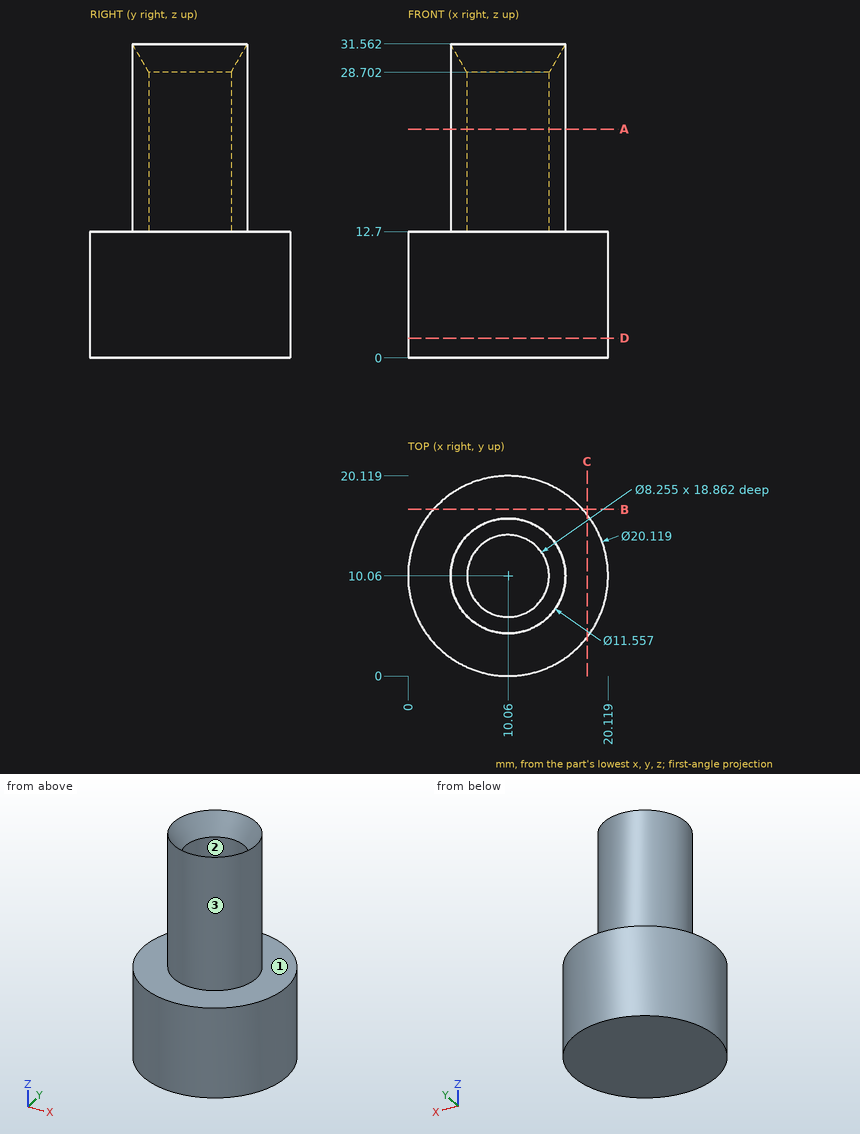
Geometry check sheet. Reference: drawing and pictorial views, mm from the part's lowest x, y, z. Round coordinates to 2 decimals unless told otherwise and drop trailing zeros. Loops run counter-clockwise (first coordinate to the right, second up) from the corner with the lowest first, then second, coordinate; pieces in that order, holes last. Notation, with made-up numbers: (44, 27.25) -> (56, 27.25) arc R33 cw to (56, 58.25) -> close; hole circle Ø9 at (-5, 19.25). An arc over 180 degrees is marked (long way). Use a Markdown table: item, result.
(1) Sectioned sample at B-B (y = 16.75). Enter the section's corners in (x, z), then the cut area to 3 significant figures.
Calculated:
| item | result |
|---|---|
| outline | (2.55, 0) -> (17.57, 0) -> (17.57, 12.7) -> (2.55, 12.7) -> close |
| area | 191 mm² |
(2) Go/stop test with flat-tipped pins: P1, Ø6.5, axis at x = 11, y = 8, coming from the +Z side (1 decimal); P2, Ø1, axis at y = 13, z = 20.5, coming from the -X side; P3, Ø2, axis at y = 5.5, z = 7, coming from the +X side. Record where each tip stops, or that it passes through.
Calculated:
| item | result |
|---|---|
| P1 | z = 31.1 |
| P2 | x = 4.82 |
| P3 | x = 19.47 |
(3) Sectioned sample at A-A (z = 23). Enter the section's corners in (x, y) (1 decimal).
Calculated:
| item | result |
|---|---|
| outline | circle Ø11.6 at (10.1, 10.1); hole circle Ø8.3 at (10.1, 10.1) |
(4) Scan lines: probe 1 along Z at (x, y) = (5.5, 1.25); probe 2 along Y at (x, z) = (8.25, 23); probe 3 along X at (y, z) = (7.25, 25.5) (1 decimal). Record each from-to range of solid material in increasing order.
Calculated:
| item | result |
|---|---|
| probe 1 | 0 to 12.7 |
| probe 2 | 4.57 to 6.35, 13.77 to 15.55 |
| probe 3 | 5 to 7, 13.1 to 15.1 |
(5) Mould release check, pull along Y, two halves, no side actions. Record for the marked faces 1, 2 and 3: released by +Y, released by -Y, zero draft, split by the parting line, or undercut.
Calculated:
| item | result |
|---|---|
| face 1 | zero draft |
| face 2 | undercut |
| face 3 | split by the parting line |
(6) Sectioned sample at D-D (z = 2). Enter the section's corners in (x, y).
Calculated:
| item | result |
|---|---|
| outline | circle Ø20.12 at (10.06, 10.06) |
(7) Sectioned sample at C-C (x = 18). Enter the section's corners in (y, z) (1 decimal).
Calculated:
| item | result |
|---|---|
| outline | (3.9, 0) -> (16.2, 0) -> (16.2, 12.7) -> (3.9, 12.7) -> close |
